Part model, mm, in its own coordinate system. Face numbers are marked on the shaded views. A direction names the side the tool comes from. Coordinates: 2 decimals unless noted, no trailing zeros. Order: outer loops, then holes, each group sorted by start corner. A loop starts at its lowest first (then second) coordinate and runs counter-clockwise, first axis right, second up.
1) Pin check, flat tips, straight feed: pin 1 Ø3.5 at (x, z) = (37, -22.68) entering from +Y; pin 2 Ø10.5 at (x, z) = (22, 51) entering from -Y; pin 3 Ø12 at (x, y) = (-10.5, 7.5) entering from -Z. Stop position of each tip, or through.
2) Cut at B-B (y = 13). List the corners of the cut face in (x, z), and give its area (3 significant figures).
3) Mould opens along Z. For the marked faces 1, 2 and 3 say: +Z half, -Z half, draft (parallel to the pull), parting line (faces both ways), or undercut.
4) Cut at C-C (y = -21). List the corners of the cut face in (x, z), and give its area (3 significant figures).
5) Wall check: L1, parallel to X at y = 7, z = 0; L2, parallel to X at y = 7, z = 14; L3, parallel to Z at x = 28.5, y = 8. Give the ranges that are in metal, low to high.
6) Tool access for the marked faces 4, 5, 6 and 7: list every direction of +Z, -Z, +X, -X, +Y, -Y with a clear straight run to the whole face (end or side of a thin tool).
```python
from build123d import *
from build123d.topology import SkipClean

# Parameters (mm, degrees)
BOSS_EXTRUDE2_DEPTH = 3
SKETCH3_R           = 4.8
BOSS_EXTRUDE3_DEPTH = 7.4
SKETCH6_R           = 16
BOSS_EXTRUDE6_DEPTH = 25
SKETCH4_R           = 38.5
BOSS_EXTRUDE4_DEPTH = 6
SKETCH5_R           = 28.2
BOSS_EXTRUDE5_DEPTH = 1.4
CHAMFER1_SIZE       = 1.4
FILLET2_R           = 2
SKETCH7_R           = 3.25
CUT_EXTRUDE1_DEPTH  = 2
CHAMFER2_SIZE       = 0.5
SKETCH9_R           = 1.5
CUT_EXTRUDE2_DEPTH  = 86.464847
BOSS_EXTRUDE7_DEPTH = 8
CUT_EXTRUDE3_START  = -6
SKETCH14_R          = 3.25
CUT_EXTRUDE3_DEPTH  = 6
SKETCH15_R          = 39
BOSS_EXTRUDE8_DEPTH = 26
FILLET3_R           = 2


with BuildPart() as part:
    # Sketch1 → Boss-Extrude2 (new body)
    with BuildSketch(Plane(origin=(0, 0, 0), x_dir=(1, 0, 0), z_dir=(0, 1, 0))):
        with BuildLine():
            ThreePointArc((26.12441, -52.949401), (0, -67.8), (-26.12441, -52.949401))
            ThreePointArc((-26.12441, -52.949401), (-35.050657, -37.22281), (-43.31697, -21.139539))
            ThreePointArc((-43.31697, -21.139539), (-40.878881, 25.537367), (0, 48.2))
            ThreePointArc((0, 48.2), (40.878881, 25.537367), (43.31697, -21.139539))
            ThreePointArc((43.31697, -21.139539), (35.050657, -37.22281), (26.12441, -52.949401))
        make_face()
    extrude(amount=BOSS_EXTRUDE2_DEPTH)

    # Sketch3 → Boss-Extrude3 (add)
    with BuildSketch(Plane.XZ):
        with Locations(Location((37, -22.683915, 0), (0, 0, 328.488032))):
            Circle(SKETCH3_R)
        with Locations(Location((-37, -22.683915, 0), (0, 0, 211.511188))):
            Circle(SKETCH3_R)
        with Locations(Location((-22, 50.49395, 0), (0, 0, 149.232316))):
            Circle(SKETCH3_R)
        with Locations(Location((22, 50.49395, 0), (0, 0, 30.76691))):
            Circle(SKETCH3_R)
    extrude(amount=BOSS_EXTRUDE3_DEPTH)

    # Sketch6 → Boss-Extrude6 (add)
    with BuildSketch(Plane.XZ):
        with Locations(Location((0, 51.8, 0), (0, 0, 89.999706))):
            Circle(SKETCH6_R)
    extrude(amount=BOSS_EXTRUDE6_DEPTH)

    # Sketch4 → Boss-Extrude4 (add)
    with BuildSketch(Plane.XZ):
        Circle(SKETCH4_R)
    extrude(amount=BOSS_EXTRUDE4_DEPTH)

    # Sketch5 → Boss-Extrude5 (add)
    with BuildSketch(Plane.XZ.offset(6)):
        with Locations(Location((0, 0, 0), (0, 0, 270))):
            Circle(SKETCH5_R)
    extrude(amount=BOSS_EXTRUDE5_DEPTH)

    # Chamfer1
    chamfer1_edges = [part.edges().sort_by_distance(p)[0] for p in [
        (0, -7.4, 28.2),
    ]]
    chamfer(chamfer1_edges, length=CHAMFER1_SIZE - 0.0001)  # a hair under: the kernel refuses the full size

    # Fillet2
    fillet2_edges = [part.edges().sort_by_distance(p)[0] for p in [
        (0, -6, -38.5),
    ]]
    fillet(fillet2_edges, radius=FILLET2_R)

    # Sketch7 → Cut-Extrude1 (cut)
    with BuildSketch(Plane.XZ.offset(7.4)):
        with Locations(Location((37, -22.683915, 0), (0, 0, 270))):
            Circle(SKETCH7_R)
        with Locations(Location((-37, -22.683915, 0), (0, 0, 270))):
            Circle(SKETCH7_R)
        with Locations(Location((-22, 50.49395, 0), (0, 0, 270))):
            Circle(SKETCH7_R)
        with Locations(Location((22, 50.49395, 0), (0, 0, 270))):
            Circle(SKETCH7_R)
    extrude(amount=-CUT_EXTRUDE1_DEPTH, mode=Mode.SUBTRACT)

    # Chamfer2
    chamfer2_edges = [part.edges().sort_by_distance(p)[0] for p in [
        (37, -7.4, -19.433915),
        (-37, -7.4, -19.433915),
        (-22, -7.4, 53.74395),
        (22, -7.4, 53.74395),
    ]]
    chamfer(chamfer2_edges, length=CHAMFER2_SIZE)

    # Sketch9 → Cut-Extrude2 (cut, through all)
    with BuildSketch(Plane.XZ.offset(5.4)):
        with Locations(Location((22, 50.49395, 0), (0, 0, 270))):
            Circle(SKETCH9_R)
        with Locations(Location((-22, 50.49395, 0), (0, 0, 270))):
            Circle(SKETCH9_R)
        with Locations(Location((-37, -22.683915, 0), (0, 0, 270))):
            Circle(SKETCH9_R)
        with Locations(Location((37, -22.683915, 0), (0, 0, 270))):
            Circle(SKETCH9_R)
    extrude(amount=-CUT_EXTRUDE2_DEPTH, mode=Mode.SUBTRACT)

    # Sketch10 → Boss-Extrude7 (add)
    with SkipClean():  # the faces are left unmerged after this step: merging them gives an invalid solid
        with BuildSketch(Plane(origin=(0, 3, 0), x_dir=(1, 0, 0), z_dir=(0, 1, 0))):
            with BuildLine():
                ThreePointArc((0, 48.2), (-40.878881, 25.537367), (-43.31697, -21.139539))
                ThreePointArc((-43.31697, -21.139539), (-35.050657, -37.22281), (-26.12441, -52.949401))
                ThreePointArc((-26.12441, -52.949401), (0, -67.8), (26.12441, -52.949401))
                ThreePointArc((26.12441, -52.949401), (35.050657, -37.22281), (43.31697, -21.139539))
                ThreePointArc((43.31697, -21.139539), (40.878881, 25.537367), (0, 48.2))
            make_face()
            with BuildLine():
                ThreePointArc((41.968932, -20.481669), (33.731063, -36.509597), (24.835532, -52.182073))
                ThreePointArc((24.835532, -52.182073), (0, -66.3), (-24.835532, -52.182073))
                ThreePointArc((-24.835532, -52.182073), (-33.731063, -36.509597), (-41.968932, -20.481669))
                ThreePointArc((-41.968932, -20.481669), (0, 46.7), (41.968932, -20.481669))
            make_face(mode=Mode.SUBTRACT)
        extrude(amount=BOSS_EXTRUDE7_DEPTH)

    # Sketch14 → Cut-Extrude3 (cut)
    with SkipClean():  # the faces are left unmerged after this step: merging them gives an invalid solid
        with BuildSketch(Plane(origin=(0, 3, 0), x_dir=(1, 0, 0), z_dir=(0, 1, 0)).offset(CUT_EXTRUDE3_START)):
            with Locations(Location((-37, 22.683915, 0), (0, 0, 90))):
                Circle(SKETCH14_R)
            with Locations(Location((37, 22.683915, 0), (0, 0, 90))):
                Circle(SKETCH14_R)
            with Locations(Location((22, -50.49395, 0), (0, 0, 90))):
                Circle(SKETCH14_R)
            with Locations(Location((-22, -50.49395, 0), (0, 0, 90))):
                Circle(SKETCH14_R)
        extrude(amount=CUT_EXTRUDE3_DEPTH, mode=Mode.SUBTRACT)

    # Sketch15 → Boss-Extrude8 (add)
    with SkipClean():  # the faces are left unmerged after this step: merging them gives an invalid solid
        with BuildSketch(Plane(origin=(0, 3, 0), x_dir=(1, 0, 0), z_dir=(0, 1, 0))):
            with Locations(Location((0, 0, 0), (0, 0, 90))):
                Circle(SKETCH15_R)
        extrude(amount=BOSS_EXTRUDE8_DEPTH)

    # Fillet3
    fillet3_edges = [part.edges().sort_by_distance(p)[0] for p in [
        (0, 29, 39),
    ]]
    fillet(fillet3_edges, radius=FILLET3_R)


solid = part.part
```
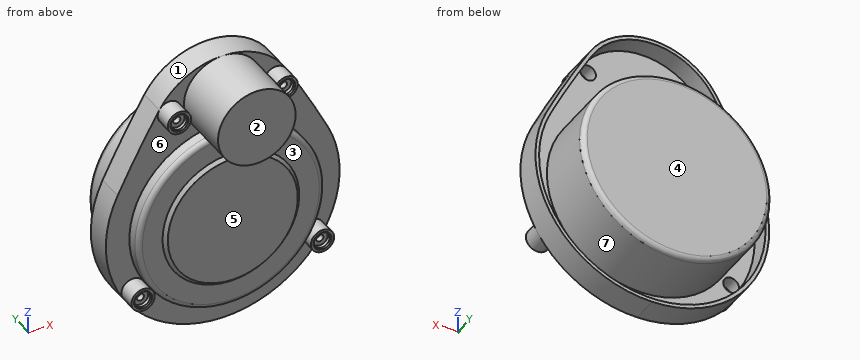
Geometry check:
1. pin 1: stops at y = -3
1. pin 2: stops at y = -7.4
1. pin 3: stops at z = -47.99
2. outline: circle Ø78 at (0, 0)
2. area: 4,780 mm2
3. face 1: +Z half
3. face 2: draft
3. face 3: undercut
4. outline: circle Ø32 at (0, 51.8)
4. area: 804 mm2
5. L1: x = -48.2 to -46.7, -39 to 39, 46.7 to 48.2
5. L2: x = -46.12 to -44.55, -36.4 to 36.4, 44.55 to 46.12
5. L3: z = -38.87 to -37, -26.62 to 26.62, 45.91 to 48.91
6. face 4: +Z, -Z, +X, -X, +Y
6. face 5: -Z, +X, -X, -Y
6. face 6: -Y
6. face 7: +Y
